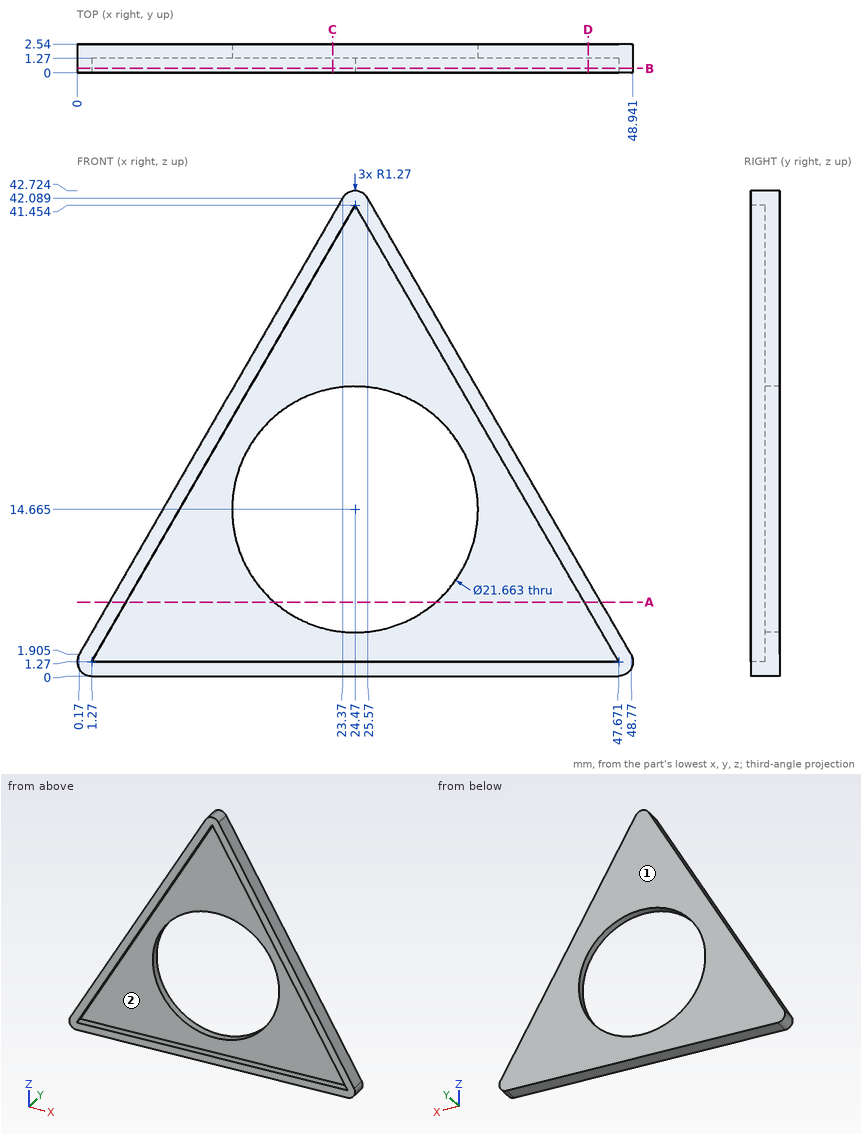
Part print with two shaded views. Sizes in mm from the minimum x, y, z corner. Coordinates: 2 decimals unless noted, no trailing zeros. Order: outer loops, then holes, each group sorted by start corner. A loop starts at its lowest first (then second) coordinate and runs counter-clockwise, first axis right, second up. Notation, with made-up numbers: M -25.75,29.25 L 24.25,29.25 A4 cw 24.25,34.25 Z; hole C 89,4 d5. An arc over 180 degrees is marked long. One line per question, with ' | ' between items. Start each with the question number.
1. Flat gauge pin, fed straight in: P1, Ø1.5, axis at y = 2, z = 22, coming from the +X side. Where does the tip first touch, or does it go through?
2. Cut at A-A (z = 6.5). Write the cut outline in (x, y).
3. Wall check: line 1 along Y through (x, z) = (17.5, 28); line 2 along X through (y, z) = (1.65, 13) (1 decimal); line 3 along X through (y, z) = (0.5, 26.5) (1 decimal). Give the ranges that are in metal, low to high. Write a range as [from, to].
4. Cut at B-B (y = 0.4). Write the cut outline in (x, z) (1 decimal), plus the area to 3 significant figures.
5. Mould opens along Z. For the marked faces 1 and 2 say: +Z half, -Z half, draft (parallel to the pull), parting line (faces both ways), or undercut.
6. Cut at C-C (x = 22.5). Write the cut outline in (y, z) (1 decimal).
7. Cut at D-D (x = 45). Write the cut outline in (y, z) (1 decimal).
The answers:
1) P1: stops at x = 37.6
2) outline: M 2.82,0 L 4.29,0 L 4.29,1.27 L 17.35,1.27 L 17.35,2.54 L 2.82,2.54 Z; M 31.59,1.27 L 44.65,1.27 L 44.65,0 L 46.12,0 L 46.12,2.54 L 31.59,2.54 Z
3) line 1: y = [1.27, 2.54] | line 2: x = [6.6, 13.8], [35.2, 42.4] | line 3: x = [14.4, 15.8], [33.1, 34.6]
4) outline: M 0.2,1.9 A1.3 ccw 1.3,0 L 47.7,0 A1.3 ccw 48.8,1.9 L 25.6,42.1 A1.3 ccw 23.4,42.1 Z; hole M 1.3,1.3 L 47.7,1.3 L 24.5,41.5 Z | area: 182 mm2
5) face 1: draft | face 2: undercut
6) outline: M 0,0 L 2.5,0 L 2.5,4 L 1.3,4 L 1.3,1.3 L 0,1.3 Z; M 0,38 L 1.3,38 L 1.3,25.3 L 2.5,25.3 L 2.5,40.6 L 0,40.6 Z
7) outline: M 0,0 L 2.5,0 L 2.5,8.4 L 0,8.4 L 0,5.9 L 1.3,5.9 L 1.3,1.3 L 0,1.3 Z
